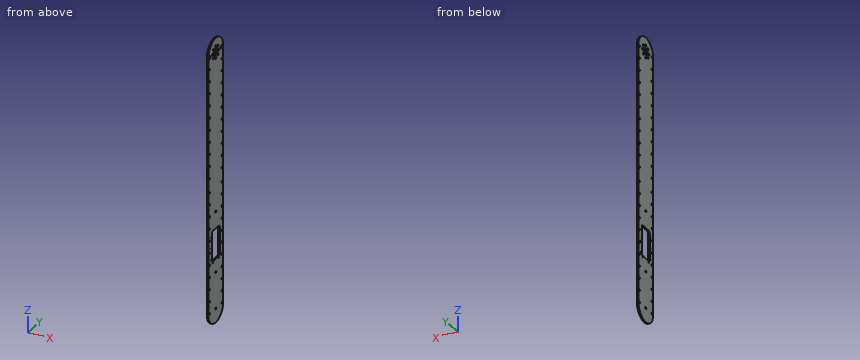
Autodesk Inventor part; units mm, degrees
ref_plane "YZ Plane" through (0, 0, 0) normal (1, 0, 0) x (0, 1, 0)
ref_plane "XZ Plane" through (0, 0, 0) normal (0, 1, 0) x (-1, 0, 0)
ref_plane "XY Plane" through (0, 0, 0) normal (0, 0, 1) x (1, 0, 0)
sketch "Sketch1" plane through (0, 0, 0) normal (1, 0, 0) x (0, 1, 0)
  line L0 (-28, 254) -> (28, 254) construction
  line L1 (28, 254) -> (28, -254)
  line L2 (28, -254) -> (-28, -254) construction
  line L3 (-28, -254) -> (-28, 254)
  line L4 (-28, 254) -> (28, -254) construction
  line L5 (28, 254) -> (-28, -254) construction
  arc A0 (28, 254) -> (-28, 254) centre (0, 254) ccw
  arc A1 (-28, -254) -> (28, -254) centre (0, -254) ccw
  circle A2 centre (0, 254) radius 7
  circle A3 centre (8.4853, 262.4853) radius 2.06
  circle A4 centre (0, 266) radius 2.06
  circle A5 centre (-8.4853, 262.4853) radius 2.06
  circle A6 centre (-12, 254) radius 2.06
  circle A7 centre (0, -254) radius 2.06
  line L6 (8.4853, 262.4853) -> (0, 254) construction
  line L7 (0, 254) -> (0, 261) construction
  circle A8 centre (-8.4853, 245.5147) radius 2.06
  circle A9 centre (0, 242) radius 2.06
  circle A10 centre (8.4853, 245.5147) radius 2.06
  circle A11 centre (12, 254) radius 2.06
  point P0 (0, 0)
  dimension "d2" = 14
  dimension "d0" = 56
  dimension "d1" = 508
  dimension "d3" = 4.12
  dimension "d8" = 360
  dimension "d10" = 4.12
  dimension "d31" = 45
  dimension "d32" = 12
extrude "Extrusion1" add sketch "Sketch1" along normal blind 3
sketch "Sketch2" plane through (3, 0, 0) normal (1, 0, 0) x (0, 0, -1)
  circle A0 centre (-254, 24) radius 2.06
  circle A1 centre (-254, 0) radius 7 construction
  line L0 (254, 28) -> (-254, 28) construction
  circle A2 centre (-230, 24) radius 2.06
  circle A3 centre (-206, 24) radius 2.06
  circle A4 centre (-182, 24) radius 2.06
  circle A5 centre (-158, 24) radius 2.06
  circle A6 centre (-134, 24) radius 2.06
  circle A7 centre (-110, 24) radius 2.06
  circle A8 centre (-86, 24) radius 2.06
  circle A9 centre (-62, 24) radius 2.06
  circle A10 centre (-38, 24) radius 2.06
  circle A11 centre (-14, 24) radius 2.06
  line L1 (0, 28) -> (0, -28) construction
  line L2 (-254, -28) -> (254, -28) construction
  arc A12 (-254, 28) -> (-254, -28) centre (-254, 0) ccw construction
  circle A13 centre (254, 0) radius 2.06 construction
  line L3 (-254, 0) -> (254, 0) construction
  circle A14 centre (254, 24) radius 2.06
  circle A15 centre (230, 24) radius 2.06
  circle A16 centre (206, 24) radius 2.06
  circle A17 centre (182, 24) radius 2.06
  circle A18 centre (158, 24) radius 2.06
  circle A19 centre (134, 24) radius 2.06
  circle A20 centre (110, 24) radius 2.06
  circle A21 centre (86, 24) radius 2.06
  circle A22 centre (62, 24) radius 2.06
  circle A23 centre (38, 24) radius 2.06
  circle A24 centre (14, 24) radius 2.06
  circle A25 centre (-254, -24) radius 2.06
  circle A26 centre (-230, -24) radius 2.06
  circle A27 centre (-206, -24) radius 2.06
  circle A28 centre (-182, -24) radius 2.06
  circle A29 centre (-158, -24) radius 2.06
  circle A30 centre (-134, -24) radius 2.06
  circle A31 centre (-110, -24) radius 2.06
  circle A32 centre (-86, -24) radius 2.06
  circle A33 centre (-62, -24) radius 2.06
  circle A34 centre (-38, -24) radius 2.06
  circle A35 centre (-14, -24) radius 2.06
  circle A36 centre (254, -24) radius 2.06
  circle A37 centre (230, -24) radius 2.06
  circle A38 centre (206, -24) radius 2.06
  circle A39 centre (182, -24) radius 2.06
  circle A40 centre (158, -24) radius 2.06
  circle A41 centre (134, -24) radius 2.06
  circle A42 centre (86, -24) radius 2.06
  circle A43 centre (62, -24) radius 2.06
  circle A44 centre (38, -24) radius 2.06
  circle A45 centre (14, -24) radius 2.06
  circle A46 centre (110, -24) radius 2.06
  point P0 (0, 0)
  dimension "d20" = 4.12
  dimension "d21" = 4
  dimension "d24" = 24
extrude "Extrusion2" cut sketch "Sketch2" against normal through all
sketch "Sketch5" plane through (3, 0, 0) normal (1, 0, 0) x (0, 0, -1)
  circle A0 centre (254, 0) radius 2.06 construction
  line L0 (254, 0) -> (110.517, 0) construction
  line L1 (110.517, 0) -> (106.517, 0) construction
  line L2 (106.517, 0) -> (106.517, -17) construction
  circle A1 centre (106.517, -17) radius 1.3
  circle A2 centre (128.517, -17) radius 1.3
  circle A3 centre (150.517, -17) radius 1.3
  circle A4 centre (106.517, 17) radius 1.3
  circle A5 centre (128.517, 17) radius 1.3
  circle A6 centre (150.517, 17) radius 1.3
  circle A7 centre (158.317, -11) radius 1.3
  circle A8 centre (158.317, 11) radius 1.3
  line L3 (152.017, -14.5) -> (99.517, -14.5) construction
  line L4 (96.017, -11) -> (96.017, 11) construction
  line L5 (99.517, 14.5) -> (152.017, 14.5) construction
  line L6 (155.517, 11) -> (155.517, -11) construction
  arc A9 (99.517, 14.5) -> (96.017, 11) centre (99.517, 11) ccw construction
  arc A10 (96.017, -11) -> (99.517, -14.5) centre (99.517, -11) ccw construction
  arc A11 (152.017, -14.5) -> (155.517, -11) centre (152.017, -11) ccw construction
  arc A12 (155.517, 11) -> (152.017, 14.5) centre (152.017, 11) ccw construction
  line L7 (95.517, 11) -> (95.517, -11)
  arc A13 (95.517, -11) -> (99.517, -15) centre (99.517, -11) ccw
  line L8 (99.517, -15) -> (152.017, -15)
  arc A14 (152.017, -15) -> (156.017, -11) centre (152.017, -11) ccw
  line L9 (156.017, -11) -> (156.017, 11)
  arc A15 (156.017, 11) -> (152.017, 15) centre (152.017, 11) ccw
  line L10 (152.017, 15) -> (99.517, 15)
  arc A16 (99.517, 15) -> (95.517, 11) centre (99.517, 11) ccw
  point P0 (0, 0)
  point P1 (155.517, -14.5)
  point P2 (96.017, 14.5)
  point P3 (155.517, 14.5)
  dimension "d37" = 143.483
  dimension "d38" = 4
  dimension "d39" = 17
  dimension "d40" = 2.6
  dimension "d41" = 2.6
  dimension "d42" = 22
  dimension "d43" = 2.6
  dimension "d44" = 22
  dimension "d45" = 2.6
  dimension "d47" = 7.8
  dimension "d48" = 11
  dimension "d49" = 14.5
  dimension "d50" = 5
  dimension "d51" = 29
  dimension "d52" = 59.5
  dimension "d53" = 3.5
  dimension "d54" = 3.5
  dimension "d55" = 0.5
extrude "Extrusion4" cut sketch "Sketch5" against normal through all
sketch "Sketch6" plane through (3, 0, 0) normal (1, 0, 0) x (0, 0, -1)
  circle A0 centre (182, 0) radius 2.06
  circle A1 centre (254, 0) radius 2.06 construction
  circle A2 centre (62, 0) radius 2.06
  point P0 (0, 0)
  dimension "d58" = 4.12
  dimension "d59" = 72
  dimension "d60" = 4.12
  dimension "d61" = 120
extrude "Extrusion5" cut sketch "Sketch6" against normal through all
hole "Hole1" at (3, 24, 254) at (3, -24, 254) direction (-1, 0, 0) diameter 4.12 end through all countersink diameter 8 countersink angle 90
equation "\"d41\" = d40"
equation "\"d43\" = d40"
properties part number "SecondStageArmBar1" material "Aluminum 6061"
Part model, mm, in its own coordinate system. Coordinates: 2 decimals unless noted, no trailing zeros. Use a Markdown table: item, result. Add a question column.
Q1. Pin check, flat tip, straight feed: P1, Ø2.5, axis at y = 0, z = -254, coming from the -X side. Stop position of the tip, or through.
Q2. Probe L1, parallel to Y at x = 1.6, z = 38; L2, parallel to Y at x = 0.65, z = -254.5; L3, parallel to Y at x = 2.1, z = -254. List the from-to ranges inside material, lowest first.
Q3. Cut at A-A (x = 1.9). Give the number of separate pieces and of enclosed holes in the cut face, and give its area (3 significant figures).
Worked out:
| question | item | result |
|---|---|---|
| 1 | P1 | passes through |
| 2 | L1 | y = -28 to -26.06, -21.94 to 21.94, 26.06 to 28 |
| 2 | L2 | y = -28 to -26, -22 to -2, 2 to 22, 26 to 28 |
| 2 | L3 | y = -28 to -26.06, -21.94 to -2.06, 2.06 to 21.94, 26.06 to 28 |
| 3 | separate pieces | 1 |
| 3 | enclosed holes | 65 |
| 3 | area | 28,200 mm2 |
